Source: CAD feature listing. Evaluate the final solid. Frame: model axes, mm. Give positions to 0.01 mm unless a question says otherwise; leave off trailing zeros. Order: outer loops, then holes, each group sorted by start corner. A loop starts at its lowest first (then second) coordinate and runs counter-clockwise, first axis right, second up.
from build123d import *

# Parameters (mm, degrees)
SKETCH1_R           = 3.5
BOSS_EXTRUDE1_DEPTH = 15
BOSS_EXTRUDE2_DEPTH = 4
SKETCH3_R           = 2.5
CUT_EXTRUDE1_DEPTH  = 108.172757733
LPATTERN1_COUNT     = 5
LPATTERN1_PITCH     = 7
BOSS_EXTRUDE3_START = 4
BOSS_EXTRUDE3_DEPTH = 4
SKETCH5_R           = 6.5
BOSS_EXTRUDE4_DEPTH = 2


with BuildPart() as part:
    # Sketch1 → Boss-Extrude1 (new body)
    with BuildSketch(Plane(origin=(0, 0, 0), x_dir=(1, 0, 0), z_dir=(0, 1, 0))):
        with Locations(Location((0, 0, 0), (0, 0, 270))):
            Circle(SKETCH1_R)
    extrude(amount=-BOSS_EXTRUDE1_DEPTH)

    # Sketch2 → Boss-Extrude2 (add)
    with BuildSketch(Plane.XZ.offset(15)):
        with BuildLine():
            Line((9.987492178, 0.5), (4.993746089, 100.25))
            ThreePointArc((4.993746089, 100.25), (0, 105), (-4.993746089, 100.25))
            Line((-4.993746089, 100.25), (-9.987492178, 0.5))
            ThreePointArc((-9.987492178, 0.5), (0, -10), (9.987492178, 0.5))
        make_face()
    extrude(amount=BOSS_EXTRUDE2_DEPTH)

    # Sketch3 → Cut-Extrude1 (cut, through all)
    with BuildSketch(Plane.XZ.offset(19)):
        with Locations(Location((0, 100, 0), (0, 0, 270))):
            Circle(SKETCH3_R)
    cut_extrude1 = extrude(amount=-CUT_EXTRUDE1_DEPTH, mode=Mode.SUBTRACT)

    # LPattern1: Cut-Extrude1 ×5
    with Locations(*[(0, 0, -i * LPATTERN1_PITCH) for i in range(1, LPATTERN1_COUNT)]):
        add(cut_extrude1, mode=Mode.SUBTRACT)

    # Sketch4 → Boss-Extrude3 (add)
    with BuildSketch(Plane(origin=(0, -15, 0), x_dir=(1, 0, 0), z_dir=(0, 1, 0)).offset(BOSS_EXTRUDE3_START)):
        with BuildLine():
            Line((-10, 0), (-10, 130))
            ThreePointArc((-10, 130), (0, 140), (10, 130))
            Line((10, 130), (10, 0))
            ThreePointArc((10, 0), (0, -10), (-10, 0))
        make_face()
        with BuildLine():
            Line((-4, 0), (-4, 130))
            ThreePointArc((-4, 130), (0, 134), (4, 130))
            Line((4, 130), (4, 0))
            ThreePointArc((4, 0), (0, -4), (-4, 0))
        make_face(mode=Mode.SUBTRACT)
    extrude(amount=-BOSS_EXTRUDE3_DEPTH)

    # Sketch5 → Boss-Extrude4 (add)
    with BuildSketch(Plane.XZ.offset(19)):
        with Locations(Location((0, 0, 0), (0, 0, 270))):
            Circle(SKETCH5_R)
    extrude(amount=BOSS_EXTRUDE4_DEPTH)


solid = part.part
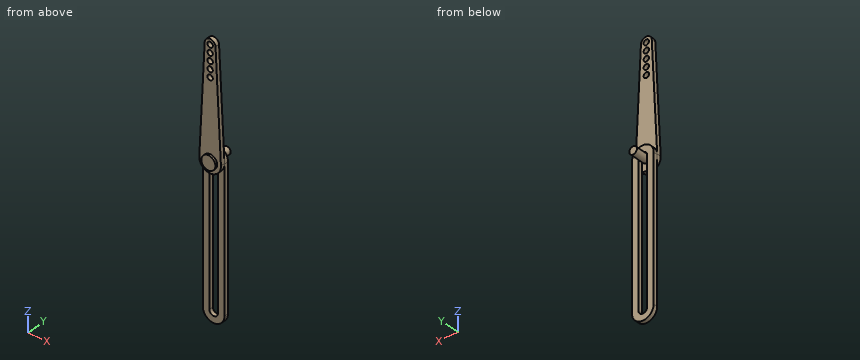
1) Section query D-D on z = 86. Output: boundary loops of the cut face in (x, y), and give its area (3 significant figures).
Checks:
outline: (-5.71, -19) - (-2.5, -19) - (-2.5, -15) - (-5.71, -15) - close; (2.5, -19) - (5.71, -19) - (5.71, -15) - (2.5, -15) - close
area: 25.7 mm2
2) Section query C-C on y = -3.5. Output: boundary loops of the cut face in (x, z), and give its area (3 significant figures).
Checks:
outline: circle Ø7 at (0, 0)
area: 38.5 mm2
3) Section query A-A on z = -32. Output: boundary loops of the cut face in (x, y).
Checks:
outline: (-10, -15) - (-4, -15) - (-4, -11) - (-10, -11) - close; (4, -15) - (10, -15) - (10, -11) - (4, -11) - close
4) Ray query, L1, parallel to X at y = -13, z = -117; L2, parallel to Y at x = 6, z = -11; L3, parallel to Y at x = -4.75, z = 36.5. Return the intervals inside material, ascending.
Checks:
L1: x = -10 to -4, 4 to 10
L2: y = -15 to -11
L3: y = -19 to -15
5) First-contact query: pin 1 Ø8 at (x, z) = (-2, -52) entering from -Y; pin 2 Ø6 at (x, z) = (2, 73.5) entering from -Y; pin 3 Ø6 at (x, z) = (2.5, 60.5) entering from +Y. Flat tips, straight axial feed; report the tip coordinate or a pass-through.
Checks:
pin 1: stops at y = -15
pin 2: stops at y = -19
pin 3: stops at y = -15
6) Section query B-B on x = 0. State how many separate pieces and enclosed holes the cut face has, and give its area (3 significant figures).
Checks:
separate pieces: 7
enclosed holes: 0
area: 539 mm2
